The listing builds one solid part. Answer for the finished solid, in the listing's coordinates (mm). Give positions to 0.01 mm unless a question says otherwise; leave off trailing zeros. Write each loop counter-clockwise with the first axis right and the second up, starting at its lowest first coordinate (ties: lowest second). Pieces come first, ordered by that corner, then holes. Notation, with made-up numbers: (42, -3) -> (71, -3) arc R22 ccw to (71, 24) -> close; hole circle Ø3 at (19, -32). An arc over 180 degrees is marked (long way). One line per question, with ' | ' between items.
from build123d import *

# Parameters (mm, degrees)
SALIENTE_EXTRUIR1_DEPTH = 0.1


with BuildPart() as part:
    # Model → Saliente-Extruir1 (new body)
    with BuildSketch(Plane.XY):
        with BuildLine():
            Line((27.419125066, -46.711901605), (17.855705746, -46.621328457))
            ThreePointArc((17.855705746, -46.621328457), (17.185424798, -46.47100647), (16.673913765, -46.012498333))
            ThreePointArc((16.673913765, -46.012498333), (16.598467504, -45.649222161), (16.794123037, -45.333975231))
            ThreePointArc((16.794123037, -45.333975231), (20.362195737, -43.279741776), (24.264393991, -41.966780746))
            ThreePointArc((24.264393991, -41.966780746), (23.908199582, -34.385858307), (23.772490147, -26.797785927))
            ThreePointArc((23.772490147, -26.797785927), (30.332057529, -28.845679283), (37.200740842, -28.638360736))
            ThreePointArc((37.200740842, -28.638360736), (36.777649791, -37.362977687), (35.226615012, -45.959037138))
            ThreePointArc((35.226615012, -45.959037138), (34.871092661, -46.500894758), (34.258012391, -46.710986181))
            Line((34.258012391, -46.710986181), (30.419140985, -46.711540389))
            Line((30.419140985, -46.711540389), (30.419140797, -42.710240543))
            Line((30.419140797, -42.710240543), (27.419140797, -42.710240543))
            Line((27.419140797, -42.710240543), (27.419125066, -46.711901605))
        make_face()
    extrude(amount=SALIENTE_EXTRUIR1_DEPTH)


solid = part.part
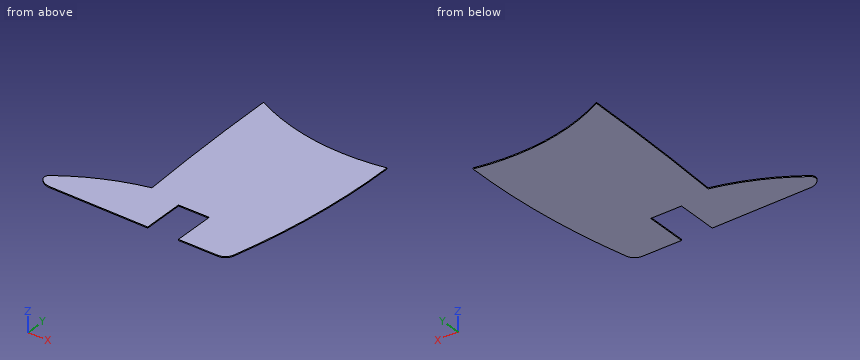
Item 1: Consider line 1 (Y direction, x = 33.5, z = 0.05); line 2 (X direction, y = -44.75, z = 0.05); line 3 (Y direction, x = 25.5, z = 0.05). Determine where each line is inside the solid, lowest interval first. Write a range as [from, to].
Answers below:
line 1: [-46.71, -29.03] | line 2: [17.65, 27.42], [30.42, 35.52] | line 3: [-46.69, -27.58]
Item 2: Find section A-A (y = -44.5). Write down the section's boundary in (x, z).
Answers below:
outline: (18.05, 0) -> (27.42, 0) -> (27.42, 0.1) -> (18.05, 0.1) -> close; (30.42, 0) -> (35.57, 0) -> (35.57, 0.1) -> (30.42, 0.1) -> close
Item 3: Find section B-B (z = 0.05). Write down the section's boundary in (x, y) (1 decimal), then the cut area to 3 significant figures.
Answers below:
outline: (16.7, -46) arc R1.4 ccw to (17.9, -46.6) -> (27.4, -46.7) -> (27.4, -42.7) -> (30.4, -42.7) -> (30.4, -46.7) -> (34.3, -46.7) arc R1 ccw to (35.2, -46) arc R67.2 ccw to (37.2, -28.6) arc R20.7 cw to (23.8, -26.8) arc R261.1 ccw to (24.3, -42) arc R20.8 ccw to (16.8, -45.3) arc R0.5 ccw to start | area: 240 mm²
Item 4: Find section C-C (y = -30). Write down the section's boundary in (x, z).
Answers below:
outline: (23.8, 0) -> (37.21, 0) -> (37.21, 0.1) -> (23.8, 0.1) -> close
Item 5: A flat-ended cylindrical pin translates along its axis: pin 1 (1.5 mm diameter, centred on x = 32.5, y = -34, fed in from -Z). Find the tip coordinate at first contact, or state that the pin passes through.
Answers below:
pin 1: z = 0
Item 6: Find section D-D (x = 25.5). Write down the section's boundary in (y, z).
Answers below:
outline: (-46.69, 0) -> (-27.58, 0) -> (-27.58, 0.1) -> (-46.69, 0.1) -> close
